from build123d import *

# Parameters (mm, degrees)
F0_W     = 11
F0_H     = 15
F1_DEPTH = 20
F3_DEPTH = 11
F5_DEPTH = 15
F7_DEPTH = 15
F9_DEPTH = 54.1


with BuildPart() as f1:
    # F0 (on Top) → F1 (new body)
    with BuildSketch(Plane.XY):
        Rectangle(F0_W, F0_H)
    extrude(amount=F1_DEPTH)

    # F2 (on face) → F3 (cut)
    with BuildSketch(Plane(origin=(-5.5, 0, 0), x_dir=(0, -1, 0), z_dir=(-1, 0, 0))):
        with BuildLine():
            ThreePointArc((0, 4), (-20.5060966544, -45.5060966544), (29, -25))
            ThreePointArc((29, -25), (20.5060966544, -4.4939033456), (0, 4))
        make_face()
    extrude(amount=-F3_DEPTH, mode=Mode.SUBTRACT)

    # F4 (on face) → F5 (join)
    with BuildSketch(Plane(origin=(-5.5, 0, 0), x_dir=(0, -1, 0), z_dir=(-1, 0, 0))):
        with BuildLine():
            Line((0, 20), (-7.5, 20))
            Line((-7.5, 20), (-7.5, 3.0133896557))
            ThreePointArc((-7.5, 3.0133896557), (-3.7823074958, 3.7522894742), (0, 4))
            Line((0, 4), (0, 20))
        make_face()
        with BuildLine():
            Line((7.5, 20), (0, 20))
            Line((0, 20), (0, 4))
            ThreePointArc((0, 4), (3.7823074958, 3.7522894742), (7.5, 3.0133896557))
            Line((7.5, 3.0133896557), (7.5, 20))
        make_face()
        with BuildLine():
            ThreePointArc((0, 4), (-3.7823074958, 3.7522894742), (-7.5, 3.0133896557))
            Line((-7.5, 3.0133896557), (-7.5, -0.105221431))
            ThreePointArc((-7.5, -0.105221431), (-3.7904984636, 0.7222106631), (0, 1))
            Line((0, 1), (0, 4))
        make_face()
        with BuildLine():
            ThreePointArc((7.5, 3.0133896557), (3.7823074958, 3.7522894742), (0, 4))
            Line((0, 4), (0, 1))
            ThreePointArc((0, 1), (3.7904984636, 0.7222106631), (7.5, -0.105221431))
            Line((7.5, -0.105221431), (7.5, 3.0133896557))
        make_face()
    extrude(amount=F5_DEPTH)

    # F6 (on face) → F7 (join)
    with BuildSketch(Plane.YZ.offset(5.5)):
        with BuildLine():
            Line((0, 20), (-7.5, 20))
            Line((-7.5, 20), (-7.5, 3.0133896557))
            ThreePointArc((-7.5, 3.0133896557), (-3.7823074958, 3.7522894742), (0, 4))
            Line((0, 4), (0, 20))
        make_face()
        with BuildLine():
            ThreePointArc((0, 4), (-3.7823074958, 3.7522894742), (-7.5, 3.0133896557))
            Line((-7.5, 3.0133896557), (-7.5, 1.9768419204))
            ThreePointArc((-7.5, 1.9768419204), (-3.7847342197, 2.7430313211), (0, 3))
            Line((0, 3), (0, 4))
        make_face()
        with BuildLine():
            ThreePointArc((7.5, 3.0133896557), (3.7823074958, 3.7522894742), (0, 4))
            Line((0, 4), (0, 3))
            ThreePointArc((0, 3), (3.7847342197, 2.7430313211), (7.5, 1.9768419204))
            Line((7.5, 1.9768419204), (7.5, 3.0133896557))
        make_face()
        with BuildLine():
            Line((7.5, 20), (0, 20))
            Line((0, 20), (0, 4))
            ThreePointArc((0, 4), (3.7823074958, 3.7522894742), (7.5, 3.0133896557))
            Line((7.5, 3.0133896557), (7.5, 20))
        make_face()
    extrude(amount=F7_DEPTH)

    # F8 (on face) → F9 (cut)
    with BuildSketch(Plane.YZ.offset(20.5)):
        with BuildLine():
            ThreePointArc((0, 12), (17.6776695297, 19.3223304703), (25, 37))
            ThreePointArc((25, 37), (-17.6776695297, 54.6776695297), (0, 12))
        make_face()
    extrude(amount=-F9_DEPTH, mode=Mode.SUBTRACT)


solid = f1.part
The listing builds one solid part. Answer for the finished solid, in the listing's coordinates (mm). Give positions to 0.01 mm unless a question says otherwise; leave off trailing zeros. Write each loop counter-clockwise with the first axis right and the second up, starting at its lowest first coordinate (ties: lowest second). Pieces come first, ordered by that corner, then holes.
Item 1: Flat-ended cylindrical pins translate along their axes: P1, Ø6, axis at x = -10.5, y = 5, coming from the -Z side; P2, Ø5, axis at x = -1, y = -3.5, coming from the +Z side; P3, Ø1.5, axis at x = 7.5, y = 2.5, coming from the +Z side. Find the tip coordinate at first contact, or state that the pin passes through.
Item 2: Section D-D, the plane x = -11 is taken. Write down the section's boundary in (y, z).
Item 3: Section A-A, the plane z = 2.5 is taken. Write down the section's boundary in (x, y).
Item 4: Determine the mould class of faces 1 (the flat face through (0, -7.5, 7)), 2 (the flat face through (-20.5, 0, 7)), 3 (the flat face through (5.5, -0.1, 3.2)), 4 (the flat face through (-5.5, 0, 2)) for opening direction Y: released by +Y, released by -Y, zero draft, split by the parting line, or undercut.
Item 5: Find the intervals of material crossed by line 1 along X through (y, z) = (-1.5, 3); line 2 along X through (y, z) = (5.75, 0.5); line 3 along Z through (x, y) = (-17, 0.25), in increasing order.
Item 6: Section C-C, the plane y = -3.5 is taken. Write down the section's boundary in (x, z).
Item 7: Section B-B, the plane x = 0 is taken. Write down the section's boundary in (y, z).
Completed:
1. P1: stops at z = -0.11
1. P2: stops at z = 12.73
1. P3: stops at z = 12.21
2. outline: (-7.5, -0.11) arc R26 cw to (7.5, -0.11) - (7.5, 13.15) arc R25 cw to (-7.5, 13.15) - close
3. outline: (-20.5, -7.5) - (-5.5, -7.5) - (-5.5, 7.5) - (-20.5, 7.5) - close; (5.5, -7.5) - (20.5, -7.5) - (20.5, -5.27) - (5.5, -5.27) - close; (5.5, 5.27) - (20.5, 5.27) - (20.5, 7.5) - (5.5, 7.5) - close
4. face 1: released by -Y
4. face 2: zero draft
4. face 3: undercut
4. face 4: undercut
5. line 1: x = -20.5 to -5.5, 5.5 to 20.5
5. line 2: x = -20.5 to -5.5
5. line 3: z = 1 to 12
6. outline: (-20.5, 0.76) - (-5.5, 0.76) - (-5.5, 3.79) - (5.5, 3.79) - (5.5, 2.78) - (20.5, 2.78) - (20.5, 12.25) - (-20.5, 12.25) - close
7. outline: (-7.5, 3.01) arc R29 cw to (7.5, 3.01) - (7.5, 13.15) arc R25 cw to (-7.5, 13.15) - close
